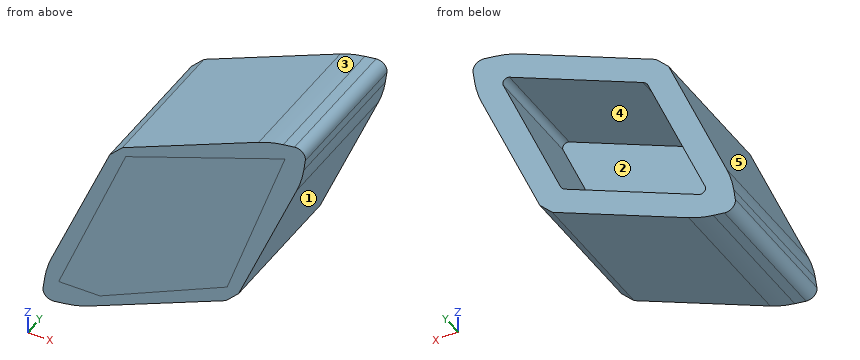
```python
from build123d import *

# Parameters (mm, degrees)
BOSS_EXTRUDE1_DEPTH = 15
BOSS_EXTRUDE2_START = -4
BOSS_EXTRUDE2_DEPTH = 4.000012


with BuildPart() as part:
    # Sketch1 → Boss-Extrude1 (new body)
    with BuildSketch(Plane(origin=(0, 0, 0), x_dir=(1, 0, 0), z_dir=(0, 1, 0))):
        with BuildLine():
            Line((-33.248720492, 21.52614432), (-19.029308571, 15.44140741))
            Line((-19.029308571, 15.44140741), (-17.714430818, 14.126529658))
            Line((-17.714430818, 14.126529658), (-11.629693909, -0.092882264))
            ThreePointArc((-11.629693909, -0.092882264), (-11.188945491, -1.347659996), (-10.918602777, -2.649827859))
            Line((-10.918602777, -2.649827859), (-10.755160033, -3.825322261))
            ThreePointArc((-10.755160033, -3.825322261), (-11.038524889, -4.670145906), (-11.883348535, -4.953510763))
            Line((-11.883348535, -4.953510763), (-13.058842937, -4.790068018))
            ThreePointArc((-13.058842937, -4.790068018), (-14.361010799, -4.519725304), (-15.615788532, -4.078976887))
            Line((-15.615788532, -4.078976887), (-29.835200454, 2.005760022))
            Line((-29.835200454, 2.005760022), (-31.150078206, 3.320637775))
            Line((-31.150078206, 3.320637775), (-37.234815116, 17.540049697))
            ThreePointArc((-37.234815116, 17.540049697), (-37.675563533, 18.794827429), (-37.945906247, 20.096995292))
            Line((-37.945906247, 20.096995292), (-38.109348992, 21.272489694))
            ThreePointArc((-38.109348992, 21.272489694), (-37.825984135, 22.117313339), (-36.98116049, 22.400678196))
            Line((-36.98116049, 22.400678196), (-35.805666088, 22.237235451))
            ThreePointArc((-35.805666088, 22.237235451), (-34.503498225, 21.966892737), (-33.248720492, 21.52614432))
        make_face()
        with BuildLine():
            Line((-34.972142842, 18.607085072), (-29.009288651, 4.672500679))
            ThreePointArc((-29.009288651, 4.672500679), (-28.797032907, 4.358805321), (-28.48333755, 4.146549578))
            Line((-28.48333755, 4.146549578), (-14.548753156, -1.816304613))
            ThreePointArc((-14.548753156, -1.816304613), (-13.998494054, -1.710176742), (-13.892366182, -1.159917639))
            Line((-13.892366182, -1.159917639), (-19.855220374, 12.774666754))
            ThreePointArc((-19.855220374, 12.774666754), (-20.067476117, 13.088362112), (-20.381171475, 13.300617855))
            Line((-20.381171475, 13.300617855), (-34.315755868, 19.263472046))
            ThreePointArc((-34.315755868, 19.263472046), (-34.86601497, 19.157344174), (-34.972142842, 18.607085072))
        make_face(mode=Mode.SUBTRACT)
    extrude(amount=BOSS_EXTRUDE1_DEPTH)

    # Sketch2 → Boss-Extrude2 (add)
    with BuildSketch(Plane.XZ.offset(BOSS_EXTRUDE2_START)):
        Polygon((-12.865216707, 3.215805982), (-29.492692689, -2.90528144), (-36.484014197, -19.947497419), (-32.173846311, -19.947497419), (-18.909952053, -13.83296991), align=None)
    extrude(amount=BOSS_EXTRUDE2_DEPTH)


solid = part.part
```
Geometry: final body of the model. Coordinates: model frame, mm. Face numbers are marked on the shaded views. A direction names the side the tool comes from. Round coordinates to 2 decimals unless told otherwise and drop trailing zeros. Order: outer loops, then holes, each group sorted by start corner. A loop starts at its lowest first (then second) coordinate and runs counter-clockwise, first axis right, second up. Notation, with made-up numbers: (47.5, 3.25) -> (68.5, 3.25) arc R23 ccw to (68.5, 38.25) -> close; hole circle Ø10 at (2.5, 59). An arc over 180 degrees is marked (long way). Use one line per item in the form item = value. Start each with the question number.
1. Draft query along X for the marked faces 1, 2 and 3. Return one class per face: pulls with the +X half, pulls with the -X half, needs draft (parallel to the pull), parting line crosses it, or undercut.
2. Reachability of the marked faces 4 and 5 from +Z, -Z, +X, -X, +Y, -Y: full face, straight path, thin tool, end or side. Return the list, or none.
3. Line query: probe 1 along Y at (x, z) = (-28.5, -9.25); probe 2 along X at (y, z) = (8.75, -18); probe 3 along X at (y, z) = (5, -8.5). Output: solid intervals per line, ascending.
4. Cut plane A-A (y = 7.25). Return the cut outline in (x, z).
5. Cut plane B-B (y = 1). Return the cut outline in (x, z).
6. Pin query (flat end, axial travel): pin 1 Ø5 at (y, z) = (7, -3.5) entering from +X; pin 2 Ø3 at (x, y) = (-18.5, 8.5) entering from +Z; pin 3 Ø2 at (y, z) = (3.5, -12.5) entering from -X; pin 4 Ø3 at (x, z) = (-17.5, -5) entering from +Y. Return the tip coordinate at first contact, or that it passes through.
Solution:
q1.face_1 = pulls with the +X half
q1.face_2 = undercut
q1.face_3 = pulls with the -X half
q2.face_4 = +Y
q2.face_5 = +Z, -X, +Y, -Y
q3.probe_1 = 0 to 4
q3.probe_2 = -37.42 to -34.71, -31.36 to -25.01
q3.probe_3 = -33.37 to -30.65, -18.03 to -15.31
q4.outline = (-38.11, -21.27) arc R1 ccw to (-36.98, -22.4) -> (-35.81, -22.24) arc R10 ccw to (-33.25, -21.53) -> (-19.03, -15.44) -> (-17.71, -14.13) -> (-11.63, 0.09) arc R10 ccw to (-10.92, 2.65) -> (-10.76, 3.83) arc R1 ccw to (-11.88, 4.95) -> (-13.06, 4.79) arc R10 ccw to (-15.62, 4.08) -> (-29.84, -2.01) -> (-31.15, -3.32) -> (-37.23, -17.54) arc R10 ccw to (-37.95, -20.1) -> close; hole (-34.97, -18.61) arc R0.5 ccw to (-34.32, -19.26) -> (-20.38, -13.3) arc R1 ccw to (-19.86, -12.77) -> (-13.89, 1.16) arc R0.5 ccw to (-14.55, 1.82) -> (-28.48, -4.15) arc R1 ccw to (-29.01, -4.67) -> close
q5.outline = (-38.11, -21.27) arc R1 ccw to (-36.98, -22.4) -> (-35.81, -22.24) arc R10 ccw to (-33.25, -21.53) -> (-19.03, -15.44) -> (-17.71, -14.13) -> (-11.63, 0.09) arc R10 ccw to (-10.92, 2.65) -> (-10.76, 3.83) arc R1 ccw to (-11.88, 4.95) -> (-13.06, 4.79) arc R10 ccw to (-15.62, 4.08) -> (-29.84, -2.01) -> (-31.15, -3.32) -> (-37.23, -17.54) arc R10 ccw to (-37.95, -20.1) -> close
q6.pin_1 = -12.1
q6.pin_2 = 3.49
q6.pin_3 = -35.51
q6.pin_4 = 15
